The model under review builds one solid part; all positions refer to its coordinate system, in mm. A direction names the side the tool comes from. Round coordinates to 2 decimals unless told otherwise and drop trailing zeros. Loops run counter-clockwise (first coordinate to the right, second up) from the corner with the lowest first, then second, coordinate; pieces in that order, holes last. Notation, with made-up numbers: M 86,-26.5 L 145,-26.5 A14 ccw 145,-8.5 Z; hole C 71.5,-22.75 d7. An arc over 180 degrees is marked long. Return JSON: item names as keys, results as strings. Group by question number.
Q1. Consider section D-D (x = 66.5). State the section outline as (y, z) points.
Q2. Consider section C-C (y = -25). State the section outline as (x, z) points, and give its area (3 significant figures).
Q3. Consider section B-B (y = 1.5). State the section outline as (x, z) points, and give its area (3 significant figures).
Q4. Consider section A-A (x = 46). State the section outline as (y, z) points, and give its area (3 significant figures).
Q5. Clearance check with a flat-ended pin moving along its axis: pin 1 Ø9 at (x, y) = (82.5, -36) entering from +Z. State where the tip first meets the part, or that it passes through.
Q6. Draft analysis for pull direction Y (two halves, no side actions). For faces 3 (the face through (77.95, -36.99, 23.17)), 4 (the face through (-1, -43.653, 26)), 5 (the face through (-58.846, 29.449, 58.27)), state which applies: pulls with the +Y half, pulls with the -Y half, needs draft (parallel to the pull), parting line crosses it, or undercut.
Q7. For faces 1 (the face through (-1, 8, 0)), 2 (the face through (-40.616, 10, 51)), list the 3-axis set-ups (+Z, -Z, +X, -X, +Y, -Y) from which the entire face can be reached by the end or side of a thin tool; tool diameter is ignored.
Q8. To check wall thickness, follow line 1 along X through (y, z) = (-37, 44.5); line 2 along Z through (x, y) = (53.5, -8); line 3 along Z through (x, y) = (-69, -13). State the ranges of each line that lie inside material, in increasing order.
from build123d import *

# Parameters (mm, degrees)
F0_W           = 177.8
F0_H           = 101.6
F1_DEPTH       = 53.34
F2_W           = 95
F2_H           = 55
F3_DEPTH       = 4
F4_D           = 7
F4_CBORE_D     = 11
F4_CBORE_DEPTH = 6.35
F2_R           = 5
F5_DEPTH       = 10


with BuildPart() as f1:
    # F0 (on Top) → F1 (new body)
    with BuildSketch(Plane.XY):
        with Locations((0.284396, 7.146878)):
            Rectangle(F0_W, F0_H)
    extrude(amount=F1_DEPTH)

    # F2 (on face) → F3 (cut)
    with BuildSketch(Plane.XY.offset(53.34)):
        with Locations((6.884396, 10.446878)):
            Rectangle(F2_W, F2_H)
    extrude(amount=-F3_DEPTH, mode=Mode.SUBTRACT)

    # F4 (through all)
    with Locations(Plane.XY.offset(53.34)):
        with Locations((-80.615604, 49.946878), (-80.615604, -35.653122), (81.184396, -35.653122), (81.184396, 49.946878)):
            CounterBoreHole(F4_D / 2, F4_CBORE_D / 2, F4_CBORE_DEPTH)

    # F2 (on face) → F5 (join)
    with BuildSketch(Plane.XY.offset(53.34)):
        with Locations((-63.615604, 27.946878)):
            Circle(F2_R)
    extrude(amount=F5_DEPTH)


solid = f1.part
Values:
{
 "1": {"outline": "M -43.65,0 L 57.95,0 L 57.95,53.34 L -43.65,53.34 Z"},
 "2": {"outline": "M -88.62,0 L 89.18,0 L 89.18,53.34 L -88.62,53.34 Z", "area": "9,480 mm2"},
 "3": {"outline": "M -88.62,0 L 89.18,0 L 89.18,53.34 L 54.38,53.34 L 54.38,49.34 L -40.62,49.34 L -40.62,53.34 L -88.62,53.34 Z", "area": "9,100 mm2"},
 "4": {"outline": "M -43.65,0 L 57.95,0 L 57.95,53.34 L 37.95,53.34 L 37.95,49.34 L -17.05,49.34 L -17.05,53.34 L -43.65,53.34 Z", "area": "5,200 mm2"},
 "5": {"pin 1": "stops at z = 53.34"},
 "6": {"face 3": "undercut", "face 4": "pulls with the -Y half", "face 5": "parting line crosses it"},
 "7": {"face 1": "-Z, +X, -X, +Y, -Y", "face 2": "+Z"},
 "8": {"line 1": "x = -88.62 to -83.85, -77.39 to 77.95, 84.41 to 89.18", "line 2": "z = 0 to 49.34", "line 3": "z = 0 to 53.34"}
}
